from build123d import *

# Parameters (mm, degrees)
F0_W      = 25.4
F0_H      = 13.716
F1_DEPTH  = 16.657
F3_DEPTH  = 25.401
F5_W      = 4.5
F5_H      = 5
F4_R      = 2.25
F6_DEPTH  = 6
F7_R      = 2.25
F8_DEPTH  = 2
F9_W      = 6
F9_H      = 0.75
F10_DEPTH = 5
F11_W     = 6
F11_H     = 0.75
F12_DEPTH = 5
F13_R     = 2
F14_R     = 2
F15_DEPTH = 0.751
F16_R     = 2
F17_DEPTH = 0.751


with BuildPart() as f1:
    # F0 (on Top) → F1 (new body)
    with BuildSketch(Plane.XY):
        Rectangle(F0_W, F0_H)
    extrude(amount=F1_DEPTH)

    # F2 (on face) → F3 (cut, through all)
    with BuildSketch(Plane(origin=(-12.7, 0, 0), x_dir=(0, -1, 0), z_dir=(-1, 0, 0))):
        Polygon((-6.858, 10.657), (-0.858, 16.657), (-6.858, 16.657), align=None)
        Polygon((6.858, 16.657), (-0.5295271985, 16.657), (0.5445904681, 14.1634047031), (4.491972737, 8.7391110137), (6.858, 6.0806702822), align=None)
    extrude(amount=-F3_DEPTH, mode=Mode.SUBTRACT)

    # F5 (on face) + F4 (on face) → F6 (cut)
    with BuildSketch(Plane.XZ.offset(6.858)):
        with Locations((-10.05, 6)):
            Rectangle(F5_W, F5_H)
        with Locations((-5.05, 6)):
            Rectangle(F5_W, F5_H)
        with Locations((-0.05, 6)):
            Rectangle(F5_W, F5_H)
        with Locations((4.95, 6)):
            Rectangle(F5_W, F5_H)
        with Locations((9.95, 6)):
            Rectangle(F5_W, F5_H)
        with Locations((14.95, 6)):
            Rectangle(F5_W, F5_H)
        with Locations((19.95, 6)):
            Rectangle(F5_W, F5_H)
        with Locations((24.95, 6)):
            Rectangle(F5_W, F5_H)
        with Locations((29.95, 6)):
            Rectangle(F5_W, F5_H)
        with Locations((34.95, 6)):
            Rectangle(F5_W, F5_H)
        with Locations((39.95, 6)):
            Rectangle(F5_W, F5_H)
        with Locations((44.95, 6)):
            Rectangle(F5_W, F5_H)
    with BuildSketch(Plane(origin=(0, 6.858, 0), x_dir=(-1, 0, 0), z_dir=(0, 1, 0))):
        with Locations((9.72, 5.3285)):
            Circle(F4_R)
        with Locations((4.72, 5.3285)):
            Circle(F4_R)
        with Locations((-0.28, 5.3285)):
            Circle(F4_R)
        with Locations((-5.28, 5.3285)):
            Circle(F4_R)
        with Locations((-10.28, 5.3285)):
            Circle(F4_R)
        with Locations((-15.28, 5.3285)):
            Circle(F4_R)
        with Locations((-20.28, 5.3285)):
            Circle(F4_R)
        with Locations((-25.28, 5.3285)):
            Circle(F4_R)
        with Locations((-30.28, 5.3285)):
            Circle(F4_R)
        with Locations((-35.28, 5.3285)):
            Circle(F4_R)
        with Locations((-40.28, 5.3285)):
            Circle(F4_R)
        with Locations((-45.28, 5.3285)):
            Circle(F4_R)
    extrude(amount=-F6_DEPTH, dir=(0, -1, 0), mode=Mode.SUBTRACT)

    # F7 (on face) → F8 (cut)
    with BuildSketch(Plane(origin=(0, 8.7575, 8.7575), x_dir=(1, 0, 0), z_dir=(0, 0.7071067812, 0.7071067812))):
        with Locations((-10.05, -6.9289393488)):
            Circle(F7_R)
        with Locations((-5.05, -6.9289393488)):
            Circle(F7_R)
        with Locations((-0.05, -6.9289393488)):
            Circle(F7_R)
        with Locations((4.95, -6.9289393488)):
            Circle(F7_R)
        with Locations((9.95, -6.9289393488)):
            Circle(F7_R)
        with Locations((14.95, -6.9289393488)):
            Circle(F7_R)
        with Locations((19.95, -6.9289393488)):
            Circle(F7_R)
        with Locations((24.95, -6.9289393488)):
            Circle(F7_R)
        with Locations((29.95, -6.9289393488)):
            Circle(F7_R)
        with Locations((34.95, -6.9289393488)):
            Circle(F7_R)
        with Locations((39.95, -6.9289393488)):
            Circle(F7_R)
        with Locations((44.95, -6.9289393488)):
            Circle(F7_R)
    extrude(amount=-F8_DEPTH, mode=Mode.SUBTRACT)

    # F9 (on face) → F10 (join)
    with BuildSketch(Plane(origin=(-12.7, 0, 0), x_dir=(0, -1, 0), z_dir=(-1, 0, 0))):
        with Locations((0, 0.375)):
            Rectangle(F9_W, F9_H)
    extrude(amount=F10_DEPTH)

    # F11 (on face) → F12 (join)
    with BuildSketch(Plane.YZ.offset(12.7)):
        with Locations((0, 0.375)):
            Rectangle(F11_W, F11_H)
    extrude(amount=F12_DEPTH)

    # F13
    f13_edges = [f1.edges().sort_by_distance(p)[0] for p in [
        (-17.7, 3, 0.375),
        (-17.7, -3, 0.375),
        (17.7, -3, 0.375),
        (17.7, 3, 0.375),
    ]]
    fillet(f13_edges, radius=F13_R)

    # F14 (on face) → F15 (cut, through all)
    with BuildSketch(Plane.XY.offset(0.75)):
        with Locations((-15.24, 0)):
            Circle(F14_R)
    extrude(amount=-F15_DEPTH, mode=Mode.SUBTRACT)

    # F16 (on face) → F17 (cut, through all)
    with BuildSketch(Plane.XY.offset(0.75)):
        with Locations((15.24, 0)):
            Circle(F16_R)
    extrude(amount=-F17_DEPTH, mode=Mode.SUBTRACT)


solid = f1.part
Read the model definition and answer for the solid it produces. Units are mm, in the model's axes. A direction names the side the tool comes from. Coordinates: 2 decimals unless noted, no trailing zeros. Loops run counter-clockwise (first coordinate to the right, second up) from the corner with the lowest first, then second, coordinate; pieces in that order, holes last. Notation, with made-up numbers: (27.25, 24.5) - (80.25, 24.5) arc R31 cw to (80.25, 54.5) - close; hole circle Ø9 at (2.25, 11). An arc over 180 degrees is marked (long way). Answer in a Markdown table with one row per item.
Q1. For faces 1 (the flat face through (5, -4, 3.5)), 2 (the flat face through (0, 0, 0)), determine the directions among +Z, -Z, +X, -X, +Y, -Y from which every point of the face is accessible in a straight line to the end or side of a thin tool.
Here are the results:
| item | result |
|---|---|
| face 1 | -Y |
| face 2 | -Z, +X, -X, +Y, -Y |
Q2. Find section C-C on z = 4. Write down the section's boundary in (x, y), plus the area to 3 significant figures.
Here are the results:
| item | result |
|---|---|
| outline | (-12.7, -6.86) - (-12.3, -6.86) - (-12.3, -0.86) - (-7.8, -0.86) - (-7.8, -6.86) - (-7.3, -6.86) - (-7.3, -0.86) - (-2.8, -0.86) - (-2.8, -6.86) - (-2.3, -6.86) - (-2.3, -0.86) - (2.2, -0.86) - (2.2, -6.86) - (2.7, -6.86) - (2.7, -0.86) - (7.2, -0.86) - (7.2, -6.86) - (7.7, -6.86) - (7.7, -0.86) - (12.2, -0.86) - (12.2, -6.86) - (12.7, -6.86) - (12.7, 6.86) - (-12.7, 6.86) - close |
| area | 213 mm^2 |
Q3. Find section D-D on y = -3.5. Write down the section's boundary in (x, z), plus the area to 3 significant figures.
Here are the results:
| item | result |
|---|---|
| outline | (-12.7, 0) - (12.7, 0) - (12.7, 10.1) - (-12.7, 10.1) - close; hole (-12.3, 3.5) - (-7.8, 3.5) - (-7.8, 8.5) - (-12.3, 8.5) - close; hole (-7.3, 3.5) - (-2.8, 3.5) - (-2.8, 8.5) - (-7.3, 8.5) - close; hole (-2.3, 3.5) - (2.2, 3.5) - (2.2, 8.5) - (-2.3, 8.5) - close; hole (2.7, 3.5) - (7.2, 3.5) - (7.2, 8.5) - (2.7, 8.5) - close; hole (7.7, 3.5) - (12.2, 3.5) - (12.2, 8.5) - (7.7, 8.5) - close |
| area | 144 mm^2 |
Q4. The mould has two halves that part along X. Classify faces 3 (the cylindrical face through (17.1, -2.43, 0.38)), 4 (the flat face through (-5.082, 2.466, 12.221)), 5 (the flat face through (13, 1, 0.75)), 6 (the flat face through (0, -4, 3.5)): pulls with the +X half, pulls with the -X half, needs draft (parallel to the pull), parting line crosses it, or undercut.
Here are the results:
| item | result |
|---|---|
| face 3 | pulls with the +X half |
| face 4 | undercut |
| face 5 | needs draft |
| face 6 | undercut |
Q5. Find section A-A on x = 15.24. Write down the section's boundary in (y, z), plus the area to 3 significant figures.
Here are the results:
| item | result |
|---|---|
| outline | (-3, 0) - (-2, 0) - (-2, 0.75) - (-3, 0.75) - close; (2, 0) - (3, 0) - (3, 0.75) - (2, 0.75) - close |
| area | 1.50 mm^2 |
Q6. Straight lines are drawn through the part: line 1 along Y through (x, z) = (-15.24, 0.25); line 2 along X through (y, z) = (-3.5, 8.75); line 3 along Z through (x, y) = (-14, 2.5). For each, find the intervals that lie inside material, in ascending order. Write a range as [from, to].
Here are the results:
| item | result |
|---|---|
| line 1 | y = [-3, -2], [2, 3] |
| line 2 | x = [-12.7, 12.7] |
| line 3 | z = [0, 0.75] |
Q7. Given P1, Ø6, axis at x = 12, z = 12.5, coming from the -Y side; P2, Ø1.5, axis at y = -5.5, z = 7, coming from the -X side; P3, Ø2, axis at x = -9, z = 7, coming from the -Y side, each flat-ended and moving along its own axis, determine where each tip first touches the part or whether it passes through.
Here are the results:
| item | result |
|---|---|
| P1 | stops at y = -3.94 |
| P2 | stops at x = -12.7 |
| P3 | stops at y = -0.86 |
Q8. Find section B-B on y = 0. Write down the section's boundary in (x, z), plus the area to 3 significant figures.
Here are the results:
| item | result |
|---|---|
| outline | (-17.7, 0) - (-17.24, 0) - (-17.24, 0.75) - (-17.7, 0.75) - close; (-13.24, 0) - (13.24, 0) - (13.24, 0.75) - (12.7, 0.75) - (12.7, 15.43) - (-12.7, 15.43) - (-12.7, 0.75) - (-13.24, 0.75) - close; (17.24, 0) - (17.7, 0) - (17.7, 0.75) - (17.24, 0.75) - close |
| area | 393 mm^2 |
